Could you check a few things on this drawing? It's one solid part, dimensions in mm from its lowest x, y, z. Give positions to 0.01 mm unless a question says otherwise; leave off trailing zeros. Loops run counter-clockwise (first coordinate to the right, second up) from the corner with the lowest first, then second, coordinate; pieces in that order, holes last. Notation, with made-up numbers: (56, -28.75) - (60, -28.75) arc R11 cw to (60, -10.75) - close; hole circle Ø4 at (76.5, 5). An arc over 180 degrees is marked (long way). Write each question's results on one line, items separated by ' | '. Start each with the question number.
(1) I need wall thicknesses on line 1 (Y direction, x = 69.85, z = 3.2); line 2 (X direction, y = 20, z = 3.15) (1 decimal); line 3 (Y direction, x = 187, z = 4.45) (1 decimal). Which ranges of each line are inside material? Lowest first, please.
(2) Suppose I cut it at A-A (z = 1.95). Count the separate pieces of the cut face and the enclosed holes in it, and give its area (3 significant figures).
(3) Suppose I cut it at C-C (y = 97). Please give me the cut outline in (x, z), and give its area (3 significant figures).
(4) Suppose I cut it at B-B (x = 160.5). Please give me the cut outline in (y, z).
(5) For pin 1 (3 mm diameter, centred on x = 107.95, y = 19.05, fed in from -Z), with a flat end and sliding along its axis, tell me the tip position at first contact or that it passes through.
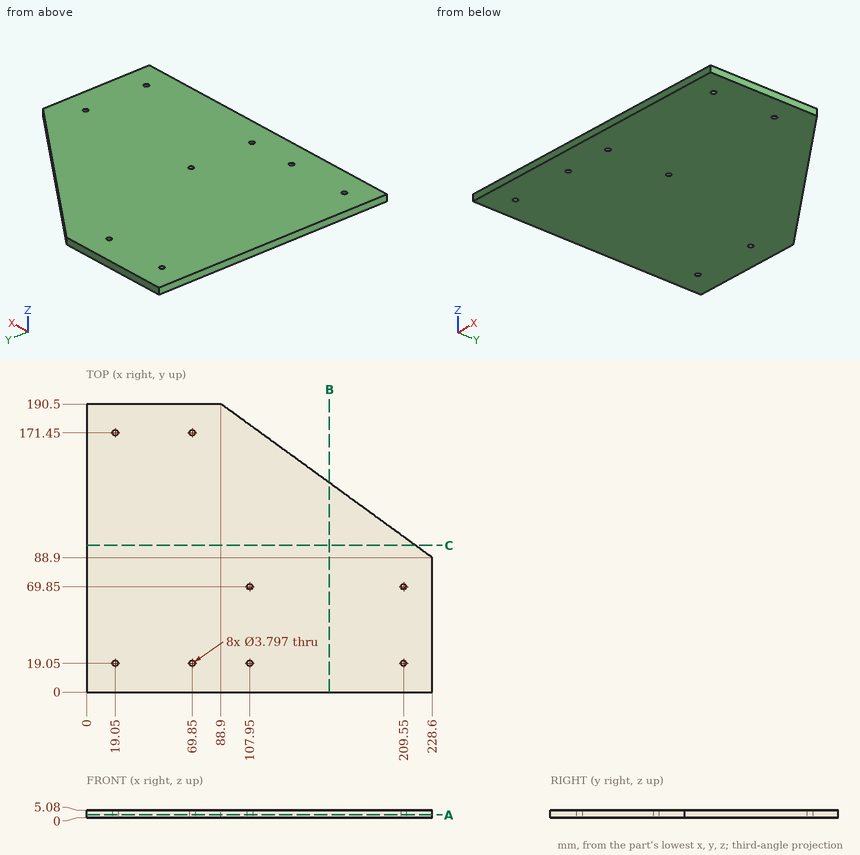
Output values:
1) line 1: 0 to 17.15, 20.95 to 169.55, 173.35 to 190.5 | line 2: 0 to 17.4, 20.7 to 68.2, 71.5 to 106.3, 109.6 to 207.9, 211.2 to 228.6 | line 3: 0 to 119.2
2) separate pieces: 1 | enclosed holes: 8 | area: 36,400 mm2
3) outline: (0, 0) - (217.46, 0) - (217.46, 5.08) - (0, 5.08) - close | area: 1,100 mm2
4) outline: (0, 0) - (138.43, 0) - (138.43, 5.08) - (0, 5.08) - close
5) pin 1: through
